```python
from build123d import *

# Parameters (mm, degrees)
F0_W     = 1900
F0_H     = 120
F1_DEPTH = 20
F2_W     = 20
F2_H     = 20
F3_DEPTH = 720
F4_W     = 150
F4_H     = 20
F5_DEPTH = 120


with BuildPart() as f1:
    # F0 (on Top) → F1 (new body)
    with BuildSketch(Plane.XY):
        with Locations((950, 60)):
            Rectangle(F0_W, F0_H)
    extrude(amount=-F1_DEPTH)

    # F2 (on face) → F3 (join)
    with BuildSketch(Plane(origin=(0, 0, -20), x_dir=(1, 0, 0), z_dir=(0, 0, -1))):
        with Locations((1890, -110)):
            Rectangle(F2_W, F2_H)
        with Locations((1890, -10)):
            Rectangle(F2_W, F2_H)
    extrude(amount=F3_DEPTH)

    # F4 (on face) → F5 (join)
    with BuildSketch(Plane(origin=(0, 120, 0), x_dir=(-1, 0, 0), z_dir=(0, 1, 0))):
        with Locations((-1805, -730)):
            Rectangle(F4_W, F4_H)
    extrude(amount=-F5_DEPTH)


solid = f1.part
```
The listing builds one solid part. Answer for the finished solid, in the listing's coordinates (mm). A direction names the side the tool comes from. Coordinates: 2 decimals unless noted, no trailing zeros. Loops run counter-clockwise (first coordinate to the right, second up) from the corner with the lowest first, then second, coordinate; pieces in that order, holes last. Notation, with made-up numbers: (76, 59) - (98, 59) arc R9 cw to (98, 72) - close; hole circle Ø3 at (68, 9.5). An arc over 180 degrees is marked (long way). Use a Markdown table: item, result. Add a question column.
1) The part is cut by section B-B, the plane y = 64. Give the vertices of the cut face in (x, z), and give its area (3 significant figures).
2) Find the intervals of material crossed by line 1 (X direction, y = 15, z = -303); line 2 (Z direction, x = 841.5, y = 63.5), in increasing order.
3) For faces 1 (the flat face through (1806, 61, -720)), 2 (the flat face through (937, 61, 0)), determine the directions among +Z, -Z, +X, -X, +Y, -Y from which every point of the face is accessible in a straight line to the end or side of a thin tool.
4) The part is cut by section C-C, the plane x = 955.5. Give the vertices of the cut face in (y, z).
5) The part is cut by section A-A, the plane z = -60. Give the vertices of the cut face in (x, y), and give its area (3 significant figures).
6) Given pin 1 (16 mm diameter, centred on y = 70.5, z = -725, fed in from -X); pin 2 (10 mm diameter, centred on y = 13.5, z = -456, fed in from -X); pin 3 (4 mm diameter, centred on x = 1421.5, y = 54, fed in from -Z), each flat-ended and moving along its own axis, determine where each tip first touches the part or whether it passes through.
Here are the results:
| question | item | result |
|---|---|---|
| 1 | outline | (0, -20) - (1900, -20) - (1900, 0) - (0, 0) - close; (1730, -740) - (1880, -740) - (1880, -720) - (1730, -720) - close |
| 1 | area | 41,000 mm^2 |
| 2 | line 1 | x = 1880 to 1900 |
| 2 | line 2 | z = -20 to 0 |
| 3 | face 1 | -X, +Y, -Y |
| 3 | face 2 | +Z, +X, -X, +Y, -Y |
| 4 | outline | (0, -20) - (120, -20) - (120, 0) - (0, 0) - close |
| 5 | outline | (1880, 0) - (1900, 0) - (1900, 20) - (1880, 20) - close; (1880, 100) - (1900, 100) - (1900, 120) - (1880, 120) - close |
| 5 | area | 800 mm^2 |
| 6 | pin 1 | stops at x = 1730 |
| 6 | pin 2 | stops at x = 1880 |
| 6 | pin 3 | stops at z = -20 |
